Could you check a few things on this model? Use its own coordinates, in mm. A direction names the side the tool comes from. Give positions to 0.01 mm unless a question says otherwise; leave off trailing zeros. Write each loop counter-clockwise with the first axis right and the second up, starting at its lowest first coordinate (ties: lowest second). Pieces come first, ordered by that corner, then holes. Notation, with made-up numbers: (-26.5, 7) - (3.5, 7) arc R31 cw to (3.5, 40) - close; hole circle Ø9 at (26, -9.5). An arc over 180 degrees is marked (long way). Write item = value, one per line.
from build123d import *

# Parameters (mm, degrees)
CROQUIS1_R                 = 1.75
SALIENTE_EXTRUIR1_DEPTH    = 11
CORTAR_EXTRUIR1_DEPTH      = 1.75
CORTAR_EXTRUIR1_DEPTH_BACK = 1.75
CROQUIS2_W                 = 0.75
CROQUIS2_H                 = 5


with BuildPart() as part:
    # Croquis1 → Saliente-Extruir1 (new body)
    with BuildSketch(Plane.XY):
        Circle(CROQUIS1_R)
    extrude(amount=SALIENTE_EXTRUIR1_DEPTH)

    # Croquis2 → Cortar-Extruir1 (cut, two sides: drawn at the far end of the back side and taken through both)
    with BuildSketch(Plane(origin=(0, 0, 0), x_dir=(1, 0, 0), z_dir=(0, 1, 0)).offset(-CORTAR_EXTRUIR1_DEPTH_BACK)):
        with Locations((-1.375, -8.5)):
            Rectangle(CROQUIS2_W, CROQUIS2_H)
        with Locations((1.375, -8.5)):
            Rectangle(CROQUIS2_W, CROQUIS2_H)
    extrude(amount=CORTAR_EXTRUIR1_DEPTH + CORTAR_EXTRUIR1_DEPTH_BACK, mode=Mode.SUBTRACT)


solid = part.part
1. For pin 1 (0.9 mm diameter, centred on y = -0.5, z = 8.5, fed in from +X), with a flat end and sliding along its axis, tell me the tip position at first contact or that it passes through.
Filled sheet:
pin_1 = 1
2. If we section it at D-D, the plane z = 5.5: Please give me the cut outline in (x, y), and give its area (3 significant figures).
Filled sheet:
outline = circle Ø3.5 at (0, 0)
area = 9.62 mm2
3. Which directions (+Z, -Z, +X, -X, +Y, -Y) give clear straight access to the entire face, cutting with the end or side of a thin tool? Please do faces 1 (the face through (1.617, -0.67, 4.201)), 2 (the face through (1, 0, 9)), 3 (the face through (-1, 0, 9)).
Filled sheet:
face_1 = +Z, -Z
face_2 = +Z, +X, +Y, -Y
face_3 = +Z, -X, +Y, -Y
4. If we section it at A-A, the plane y = -0.1: Please give me the cut outline in (x, z).
Filled sheet:
outline = (-1.75, 0) - (1.75, 0) - (1.75, 6) - (1, 6) - (1, 11) - (-1, 11) - (-1, 6) - (-1.75, 6) - close
5. I need wall thicknesses on line 1 (X direction, y = -0.3, z = 7.25); line 2 (Z direction, x = 1.1, y = -0.7); line 3 (Y direction, x = -0.45, z = 10.75). Which ranges of each line are inside material? Lowest first, please.
Filled sheet:
line_1 = -1 to 1
line_2 = 0 to 6
line_3 = -1.69 to 1.69
6. If we section it at C-C, the plane x = 0.9: Please give me the cut outline in (y, z).
Filled sheet:
outline = (-1.5, 0) - (1.5, 0) - (1.5, 11) - (-1.5, 11) - close
7. If we section it at B-B, the plane z = 9.5: Please give me the cut outline in (x, y).
Filled sheet:
outline = (-1, -1.44) arc R1.75 ccw to (1, -1.44) - (1, 1.44) arc R1.75 ccw to (-1, 1.44) - close
